Job drawing, mm, ordinate dimensions from the low corner. One solid piece. Round coordinates to 2 decimals unless told otherwise and drop trailing zeros. Write each loop counter-clockwise with the first axis right and the second up, starting at its lowest first coordinate (ties: lowest second). Pieces come first, ordered by that corner, then holes.
1) Flat gauge pins, fed straight in: pin 1 (2 mm diameter, centred on x = 22.5, z = 12.5, fed in from -Y); pin 2 (16 mm diameter, centred on x = 22.5, y = 22.5, fed in from +Z); pin 3 (5 mm diameter, centred on x = 36.5, y = 22.5, fed in from +Z). Where does each tip first touch, or does it go through?
2) Saw through at A-A (x = 22.5). Write the cut outline in (y, z).
3) Pull direction X, two halves, no side cores. Call the marked faces 1, 2 and 3: +X half, -X half, draft (parallel to the pull), parting line (faces both ways), or undercut.
4) Wall check: probe 1 along X at (y, z) = (22.5, 16.9); probe 2 along X at (y, z) = (22.5, 17.5); probe 3 along Z at (x, y) = (14, 27). Give the ranges that are in metal, low to high.
5) Saw through at B-B (z = 2). Write the cut outline in (x, y).
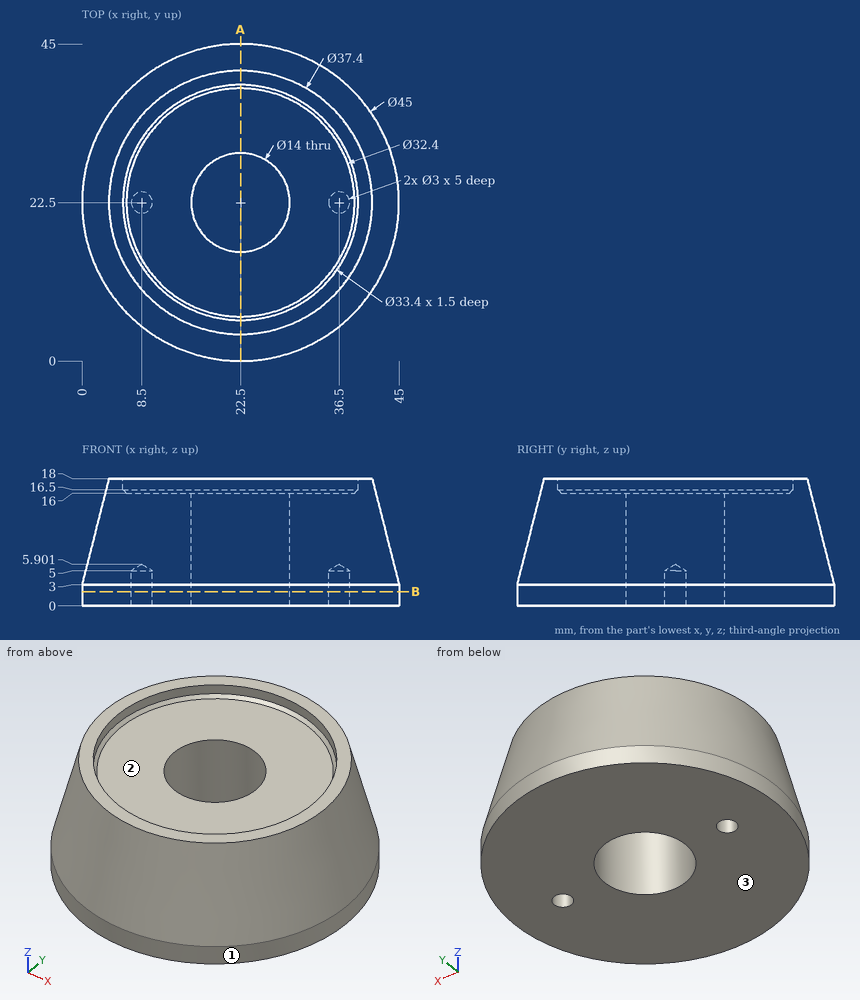
Evaluation:
1. pin 1: stops at y = 2.15
1. pin 2: stops at z = 16
1. pin 3: stops at z = 16.3
2. outline: (0, 0) - (15.5, 0) - (15.5, 16) - (6.3, 16) - (5.8, 16.5) - (5.8, 18) - (3.8, 18) - (0, 3) - close; (29.5, 0) - (45, 0) - (45, 3) - (41.2, 18) - (39.2, 18) - (39.2, 16.5) - (38.7, 16) - (29.5, 16) - close
3. face 1: parting line
3. face 2: undercut
3. face 3: draft
4. probe 1: x = 3.52 to 5.8, 39.2 to 41.48
4. probe 2: x = 3.67 to 5.8, 39.2 to 41.33
4. probe 3: z = 0 to 16
5. outline: circle Ø45 at (22.5, 22.5); hole circle Ø3 at (8.5, 22.5); hole circle Ø14 at (22.5, 22.5); hole circle Ø3 at (36.5, 22.5)
